from build123d import *

# Parameters (mm, degrees)
F0_W      = 150
F0_H      = 55
F1_DEPTH  = 2
F2_R      = 1.5
F3_DEPTH  = 2.001
F4_R      = 3
F5_DEPTH  = 25
F6_W      = 6
F6_H      = 6
F7_DEPTH  = 3.4
F8_W      = 98
F8_H      = 60
F9_DEPTH  = 4
F10_W     = 98
F10_H     = 40
F11_DEPTH = 9.2
F12_W     = 30
F12_H     = 37
F13_DEPTH = 3


with BuildPart() as f1:
    # F0 (on Front) → F1 (new body)
    with BuildSketch(Plane.XZ):
        Rectangle(F0_W, F0_H)
    extrude(amount=F1_DEPTH)

    # F2 (on face) → F3 (cut, through all)
    with BuildSketch(Plane.XZ.offset(2)):
        with Locations((-72.25, 25)):
            Circle(F2_R)
        with Locations((-72.25, -25)):
            Circle(F2_R)
        with Locations((72.25, 25)):
            Circle(F2_R)
        with Locations((72.25, -25)):
            Circle(F2_R)
    extrude(amount=-F3_DEPTH, mode=Mode.SUBTRACT)

    # F4 (on face) → F5 (join)
    with BuildSketch(Plane.XZ.offset(2)):
        with Locations((62, -2.5)):
            Circle(F4_R)
    extrude(amount=F5_DEPTH)

    # F6 (on face) → F7 (join)
    with BuildSketch(Plane.XZ.offset(2)):
        with Locations((62, -19.5)):
            Rectangle(F6_W, F6_H)
    extrude(amount=F7_DEPTH)

    # F8 (on face) → F9 (join)
    with BuildSketch(Plane.XZ.offset(2)):
        with Locations((-12.7, -6)):
            Rectangle(F8_W, F8_H)
    extrude(amount=F9_DEPTH)

    # F10 (on face) → F11 (join)
    with BuildSketch(Plane.XZ.offset(6)):
        with Locations((-12.7, -6)):
            Rectangle(F10_W, F10_H)
    extrude(amount=F11_DEPTH)

    # F12 (on face) → F13 (join)
    with BuildSketch(Plane(origin=(0, 0, 0), x_dir=(-1, 0, 0), z_dir=(0, 1, 0))):
        with Locations((-37.488226, 16)):
            Rectangle(F12_W, F12_H)
    extrude(amount=F13_DEPTH)


solid = f1.part
Model file for the job. Use its own axes, mm. A direction names the side the tool comes from. Round coordinates to 2 decimals unless told otherwise and drop trailing zeros. Loops run counter-clockwise (first coordinate to the right, second up) from the corner with the lowest first, then second, coordinate; pieces in that order, holes last. Notation, with made-up numbers: M 57,76 L 67,76 A23 ccw 67,106 Z; hole C 23.25,86.25 d11. An arc over 180 degrees is marked long. One line per question, with ' | ' between items.
1) Mould opens along X. For faces 1 (the flat face through (22.488, 1, 16)), 2 (the flat face through (59, -4, -20)), 3 (the flat face through (38, 3, 16)) say: +X half, -X half, draft (parallel to the pull), parting line (faces both ways), or undercut.
Solved:
face 1: -X half | face 2: undercut | face 3: draft
2) 3-axis set-ups, long thin cutter, end or side, ignore diameter. For faces 4 (the flat face through (38, 0, 31)), 5 (the flat face through (38, 1, -2.5)), 6 (the flat face through (36.3, -9, -6)), 7 (the flat face through (62, -5.4, -19)): which of +Z, -Z, +X, -X, +Y, -Y reach the whole face in a straight line?
Solved:
face 4: +Z, +X, -X, -Y | face 5: -Z, +X, -X, +Y | face 6: +Z, -Z, -Y | face 7: -Z, +X, -Y
3) Drill centre lines: line 1 along Z through (x, y) = (-72.25, -1.4); line 2 along Y through (x, z) = (58, 3.5); line 3 along X through (y, z) = (-7.75, 12.5). Where is each one in solid material? Low to high.
Solved:
line 1: z = -27.5 to -26.5, -23.5 to 23.5, 26.5 to 27.5 | line 2: y = -2 to 0 | line 3: x = -61.7 to 36.3
4) Band-saw the part on C-C (x = 33.5). Give the cut face in (y, z).
Solved:
outline: M -15.2,-26 L -6,-26 L -6,-36 L -2,-36 L -2,-27.5 L 0,-27.5 L 0,-2.5 L 3,-2.5 L 3,34.5 L 0,34.5 L 0,27.5 L -2,27.5 L -2,24 L -6,24 L -6,14 L -15.2,14 Z
5) Band-saw the part on A-A (x = -72.25). Give the cut face in (y, z).
Solved:
outline: M -2,-27.5 L 0,-27.5 L 0,-26.5 L -2,-26.5 Z; M -2,-23.5 L 0,-23.5 L 0,23.5 L -2,23.5 Z; M -2,26.5 L 0,26.5 L 0,27.5 L -2,27.5 Z
6) Flat gauge pins, fed straight in: pin 1 (1.8 mm diameter, centred on x = 61.5, z = -20, fed in from -Y); pin 2 (1 mm diameter, centred on y = -17.5, z = 5, fed in from -X); pin 3 (3 mm diameter, centred on x = -23.5, y = -14, fed in from -Z); pin 4 (12 mm diameter, centred on x = -12.5, y = -11, fed in from -Z). Where does each tip first touch, or does it go through?
Solved:
pin 1: stops at y = -5.4 | pin 2: passes through | pin 3: stops at z = -26 | pin 4: stops at z = -36
7) Band-saw the part on B-B (y = -3.5). Give the cut face in (x, z), then the cut area to 3 significant figures.
Solved:
outline: M -61.7,-36 L 36.3,-36 L 36.3,24 L -61.7,24 Z; M 59,-22.5 L 65,-22.5 L 65,-16.5 L 59,-16.5 Z; C 62,-2.5 d6 | area: 5,940 mm²
8) Band-saw the part on D-D (z = 21). Give the cut face in (x, y), then the cut area to 3 significant figures.
Solved:
outline: M -75,-2 L -61.7,-2 L -61.7,-6 L 36.3,-6 L 36.3,-2 L 75,-2 L 75,0 L 52.49,0 L 52.49,3 L 22.49,3 L 22.49,0 L -75,0 Z | area: 782 mm²
